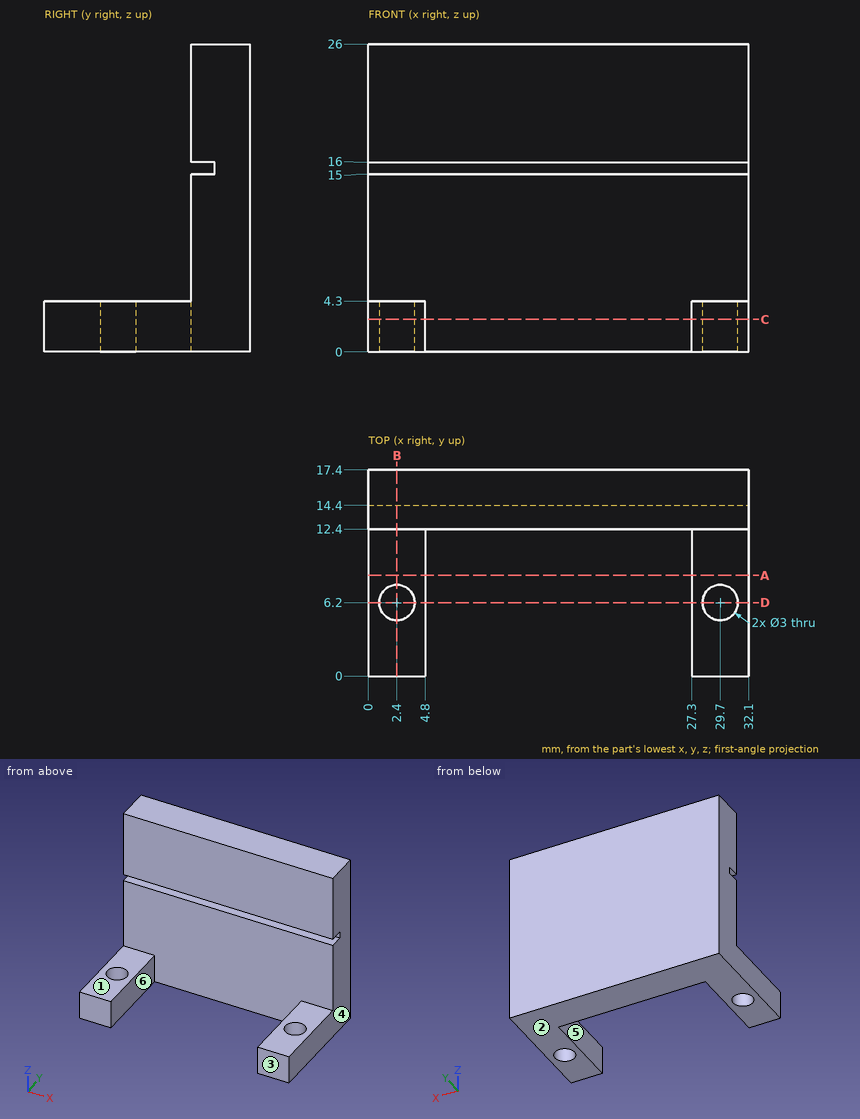
For this review, use the dimensioned drawing (mm, ordinates from the lowest corner) and the shaded views. A direction names the side the tool comes from. Coordinates: 2 decimals unless noted, no trailing zeros. Order: outer loops, then holes, each group sorted by start corner. A loop starts at its lowest first (then second) coordinate and runs counter-clockwise, first axis right, second up. Notation, with made-up numbers: M -18,-30.5 L 21,-30.5 A35 ccw 21,3.5 Z; hole C -24.5,-19.75 d10. An arc over 180 degrees is marked long. Answer as a JSON object with one key per item and string values. Group by question number.
1) Add section A-A, the plane y = 8.5. Write out the cut boundary in (x, z).
2) Wall thickness on L1, parallel to X at y = 6.2, z = 1.7; L2, parallel to Z at x = 6, y = 12.75; L3, parallel to X at y = 4.5, z = 2.5: over which ranges is each line inside the solid? List them lowest first.
3) Tool access review of the marked faces 1 and 2: name each direction out of +Z, -Z, +X, -X, +Y, -Y from which nothing blocks a thin tool from reaching the whole face with its end or side.
4) Add section C-C, the plane z = 2.75. Write out the cut boundary in (x, y), then the cut area to 3 significant figures.
5) Add section D-D, the plane y = 6.2. Write out the cut boundary in (x, z), then the cut area to 3 significant figures.
6) Mouldability with a two-part tool opening along X and no side actions: class the marked faces 3, 4, 5 and 6 as pulls with the +X half, pulls with the -X half, needs draft (parallel to the pull), parting line crosses it, or undercut.
7) Add section B-B, the plane x = 2.4. Write out the cut boundary in (y, z), then the cut area to 3 significant figures.
8) For pin 1 (6 mm diameter, centred on x = 9.5, z = 20, fed in from -Y); pin 2 (2 mm diameter, centred on y = 4, z = 3, fed in from -X); pin 3 (0.8 mm diameter, centred on x = 22, z = 15.5, fed in from -Y); pin 4 (5.5 mm diameter, centred on x = 3, y = 8.5, fed in from +Z), all flat-tipped, find the tip position at first contact; note any pin that passes through.
Computed values:
{
 "1": {"outline": "M 0,0 L 4.8,0 L 4.8,4.3 L 0,4.3 Z; M 27.3,0 L 32.1,0 L 32.1,4.3 L 27.3,4.3 Z"},
 "2": {"L1": "x = 0 to 0.9, 3.9 to 4.8, 27.3 to 28.2, 31.2 to 32.1", "L2": "z = 0 to 15, 16 to 26", "L3": "x = 0 to 4.8, 27.3 to 32.1"},
 "3": {"face 1": "+Z, +X, -X, -Y", "face 2": "-Z, +X, -X, +Y, -Y"},
 "4": {"outline": "M 0,0 L 4.8,0 L 4.8,12.4 L 27.3,12.4 L 27.3,0 L 32.1,0 L 32.1,17.4 L 0,17.4 Z; hole C 2.4,6.2 d3; hole C 29.7,6.2 d3", "area": "265 mm^2"},
 "5": {"outline": "M 0,0 L 0.9,0 L 0.9,4.3 L 0,4.3 Z; M 3.9,0 L 4.8,0 L 4.8,4.3 L 3.9,4.3 Z; M 27.3,0 L 28.2,0 L 28.2,4.3 L 27.3,4.3 Z; M 31.2,0 L 32.1,0 L 32.1,4.3 L 31.2,4.3 Z", "area": "15.5 mm^2"},
 "6": {"face 3": "needs draft", "face 4": "pulls with the +X half", "face 5": "undercut", "face 6": "undercut"},
 "7": {"outline": "M 0,0 L 4.7,0 L 4.7,4.3 L 0,4.3 Z; M 7.7,0 L 17.4,0 L 17.4,26 L 12.4,26 L 12.4,16 L 14.4,16 L 14.4,15 L 12.4,15 L 12.4,4.3 L 7.7,4.3 Z", "area": "168 mm^2"},
 "8": {"pin 1": "stops at y = 12.4", "pin 2": "stops at x = 0", "pin 3": "stops at y = 14.4", "pin 4": "stops at z = 4.3"}
}
